```python
from build123d import *

# Parameters (mm, degrees)
F1_DEPTH = 40
F2_R     = 34
F3_T     = -1
F4_DEPTH = 1


# Not quite as in the source:
# - a shell that OpenCascade refuses in one call is made with other operations: the cavity is built on its own and cut out
# - a feature names something its author has since deleted; it is built from what else it names


with BuildPart() as f1:
    # F0 (on Top) → F1 (new body)
    with BuildSketch(Plane.XY):
        with BuildLine():
            Line((37, 0.6), (39.9954997468, 0.6))
            ThreePointArc((39.9954997468, 0.6), (28.2842712475, 28.2842712475), (0.6, 39.9954997468))
            Line((0.6, 39.9954997468), (0.6, 37))
            Line((0.6, 37), (-2.4, 37))
            Line((-2.4, 37), (-2.4, 39.9279350831))
            ThreePointArc((-2.4, 39.9279350831), (-28.9139450641, 27.6402565261), (-39.9954997468, 0.6))
            Line((-39.9954997468, 0.6), (-37, 0.6))
            Line((-37, 0.6), (-37, -2.4))
            Line((-37, -2.4), (-39.9279350831, -2.4))
            ThreePointArc((-39.9279350831, -2.4), (-28.2842712475, -28.2842712475), (-2.4, -39.9279350831))
            Line((-2.4, -39.9279350831), (-2.4, -37))
            Line((-2.4, -37), (0.6, -37))
            Line((0.6, -37), (0.6, -39.9954997468))
            ThreePointArc((0.6, -39.9954997468), (27.6402565261, -28.9139450641), (39.9279350831, -2.4))
            Line((39.9279350831, -2.4), (37, -2.4))
            Line((37, -2.4), (37, 0.6))
        make_face()
        with BuildLine():
            ThreePointArc((39.9279350831, -2.4), (39.9819797116, -1.2005408523), (40, 0))
            ThreePointArc((40, 0), (39.9988749209, 0.3000084383), (39.9954997468, 0.6))
            Line((39.9954997468, 0.6), (37, 0.6))
            Line((37, 0.6), (37, -2.4))
            Line((37, -2.4), (39.9279350831, -2.4))
        make_face()
        with BuildLine():
            Line((37, 0.6), (39.9954997468, 0.6))
            ThreePointArc((39.9954997468, 0.6), (28.2842712475, 28.2842712475), (0.6, 39.9954997468))
            Line((0.6, 39.9954997468), (0.6, 37))
            Line((0.6, 37), (-2.4, 37))
            Line((-2.4, 37), (-2.4, 39.9279350831))
            ThreePointArc((-2.4, 39.9279350831), (-28.9139450641, 27.6402565261), (-39.9954997468, 0.6))
            Line((-39.9954997468, 0.6), (-37, 0.6))
            Line((-37, 0.6), (-37, -2.4))
            Line((-37, -2.4), (-39.9279350831, -2.4))
            ThreePointArc((-39.9279350831, -2.4), (-28.2842712475, -28.2842712475), (-2.4, -39.9279350831))
            Line((-2.4, -39.9279350831), (-2.4, -37))
            Line((-2.4, -37), (0.6, -37))
            Line((0.6, -37), (0.6, -39.9954997468))
            ThreePointArc((0.6, -39.9954997468), (27.6402565261, -28.9139450641), (39.9279350831, -2.4))
            Line((39.9279350831, -2.4), (37, -2.4))
            Line((37, -2.4), (37, 0.6))
        make_face()
        with BuildLine():
            Line((37, 0.6), (39.9954997468, 0.6))
            ThreePointArc((39.9954997468, 0.6), (28.2842712475, 28.2842712475), (0.6, 39.9954997468))
            Line((0.6, 39.9954997468), (0.6, 37))
            Line((0.6, 37), (-2.4, 37))
            Line((-2.4, 37), (-2.4, 39.9279350831))
            ThreePointArc((-2.4, 39.9279350831), (-28.9139450641, 27.6402565261), (-39.9954997468, 0.6))
            Line((-39.9954997468, 0.6), (-37, 0.6))
            Line((-37, 0.6), (-37, -2.4))
            Line((-37, -2.4), (-39.9279350831, -2.4))
            ThreePointArc((-39.9279350831, -2.4), (-28.2842712475, -28.2842712475), (-2.4, -39.9279350831))
            Line((-2.4, -39.9279350831), (-2.4, -37))
            Line((-2.4, -37), (0.6, -37))
            Line((0.6, -37), (0.6, -39.9954997468))
            ThreePointArc((0.6, -39.9954997468), (27.6402565261, -28.9139450641), (39.9279350831, -2.4))
            Line((39.9279350831, -2.4), (37, -2.4))
            Line((37, -2.4), (37, 0.6))
        make_face()
        with BuildLine():
            Line((37, 0.6), (39.9954997468, 0.6))
            ThreePointArc((39.9954997468, 0.6), (28.2842712475, 28.2842712475), (0.6, 39.9954997468))
            Line((0.6, 39.9954997468), (0.6, 37))
            Line((0.6, 37), (-2.4, 37))
            Line((-2.4, 37), (-2.4, 39.9279350831))
            ThreePointArc((-2.4, 39.9279350831), (-28.9139450641, 27.6402565261), (-39.9954997468, 0.6))
            Line((-39.9954997468, 0.6), (-37, 0.6))
            Line((-37, 0.6), (-37, -2.4))
            Line((-37, -2.4), (-39.9279350831, -2.4))
            ThreePointArc((-39.9279350831, -2.4), (-28.2842712475, -28.2842712475), (-2.4, -39.9279350831))
            Line((-2.4, -39.9279350831), (-2.4, -37))
            Line((-2.4, -37), (0.6, -37))
            Line((0.6, -37), (0.6, -39.9954997468))
            ThreePointArc((0.6, -39.9954997468), (27.6402565261, -28.9139450641), (39.9279350831, -2.4))
            Line((39.9279350831, -2.4), (37, -2.4))
            Line((37, -2.4), (37, 0.6))
        make_face()
        with BuildLine():
            ThreePointArc((39.9279350831, -2.4), (39.9819797116, -1.2005408523), (40, 0))
            ThreePointArc((40, 0), (39.9988749209, 0.3000084383), (39.9954997468, 0.6))
            Line((39.9954997468, 0.6), (37, 0.6))
            Line((37, 0.6), (37, -2.4))
            Line((37, -2.4), (39.9279350831, -2.4))
        make_face()
        with BuildLine():
            ThreePointArc((-2.4, -39.9279350831), (-0.9006338024, -39.989859449), (0.6, -39.9954997468))
            Line((0.6, -39.9954997468), (0.6, -37))
            Line((0.6, -37), (-2.4, -37))
            Line((-2.4, -37), (-2.4, -39.9279350831))
        make_face()
        with BuildLine():
            Line((-37, 0.6), (-39.9954997468, 0.6))
            ThreePointArc((-39.9954997468, 0.6), (-39.989859449, -0.9006338024), (-39.9279350831, -2.4))
            Line((-39.9279350831, -2.4), (-37, -2.4))
            Line((-37, -2.4), (-37, 0.6))
        make_face()
        with BuildLine():
            Line((0.6, 37), (0.6, 39.9954997468))
            ThreePointArc((0.6, 39.9954997468), (-0.9006338024, 39.989859449), (-2.4, 39.9279350831))
            Line((-2.4, 39.9279350831), (-2.4, 37))
            Line((-2.4, 37), (0.6, 37))
        make_face()
        with BuildLine():
            Line((37, 0.6), (39.9954997468, 0.6))
            ThreePointArc((39.9954997468, 0.6), (28.2842712475, 28.2842712475), (0.6, 39.9954997468))
            Line((0.6, 39.9954997468), (0.6, 37))
            Line((0.6, 37), (-2.4, 37))
            Line((-2.4, 37), (-2.4, 39.9279350831))
            ThreePointArc((-2.4, 39.9279350831), (-28.9139450641, 27.6402565261), (-39.9954997468, 0.6))
            Line((-39.9954997468, 0.6), (-37, 0.6))
            Line((-37, 0.6), (-37, -2.4))
            Line((-37, -2.4), (-39.9279350831, -2.4))
            ThreePointArc((-39.9279350831, -2.4), (-28.2842712475, -28.2842712475), (-2.4, -39.9279350831))
            Line((-2.4, -39.9279350831), (-2.4, -37))
            Line((-2.4, -37), (0.6, -37))
            Line((0.6, -37), (0.6, -39.9954997468))
            ThreePointArc((0.6, -39.9954997468), (27.6402565261, -28.9139450641), (39.9279350831, -2.4))
            Line((39.9279350831, -2.4), (37, -2.4))
            Line((37, -2.4), (37, 0.6))
        make_face()
        with BuildLine():
            Line((37, 0.6), (39.9954997468, 0.6))
            ThreePointArc((39.9954997468, 0.6), (28.2842712475, 28.2842712475), (0.6, 39.9954997468))
            Line((0.6, 39.9954997468), (0.6, 37))
            Line((0.6, 37), (-2.4, 37))
            Line((-2.4, 37), (-2.4, 39.9279350831))
            ThreePointArc((-2.4, 39.9279350831), (-28.9139450641, 27.6402565261), (-39.9954997468, 0.6))
            Line((-39.9954997468, 0.6), (-37, 0.6))
            Line((-37, 0.6), (-37, -2.4))
            Line((-37, -2.4), (-39.9279350831, -2.4))
            ThreePointArc((-39.9279350831, -2.4), (-28.2842712475, -28.2842712475), (-2.4, -39.9279350831))
            Line((-2.4, -39.9279350831), (-2.4, -37))
            Line((-2.4, -37), (0.6, -37))
            Line((0.6, -37), (0.6, -39.9954997468))
            ThreePointArc((0.6, -39.9954997468), (27.6402565261, -28.9139450641), (39.9279350831, -2.4))
            Line((39.9279350831, -2.4), (37, -2.4))
            Line((37, -2.4), (37, 0.6))
        make_face()
    extrude(amount=F1_DEPTH)

    # F2
    f2_edges = [f1.edges().sort_by_distance(p)[0] for p in [
        (-0.6, -39.9955, 40),
    ]]
    fillet(f2_edges, radius=F2_R)

    # F3: a shell. OpenCascade refuses it in one call, so the cavity is built on its own and cut out:
    # the body offset inwards by the wall thickness, plus a prism from it out through each open face.
    f3_core = offset(f1.part, amount=F3_T, mode=Mode.PRIVATE)
    f3_exits = [f3_core.faces().sort_by_distance(p)[0] for p in [
        (0, 0, 39),
        (0, 0, 1),
    ]]
    add(f3_core, mode=Mode.SUBTRACT)
    extrude(f3_exits, amount=-F3_T, mode=Mode.SUBTRACT)

    # F0 (on Top) → F4 (join)
    with BuildSketch(Plane.XY):
        with BuildLine():
            ThreePointArc((39.9279350831, -2.4), (39.9819797116, -1.2005408523), (40, 0))
            ThreePointArc((40, 0), (39.9988749209, 0.3000084383), (39.9954997468, 0.6))
            Line((39.9954997468, 0.6), (37, 0.6))
            Line((37, 0.6), (37, -2.4))
            Line((37, -2.4), (39.9279350831, -2.4))
        make_face()
        with BuildLine():
            Line((0.6, 37), (0.6, 39.9954997468))
            ThreePointArc((0.6, 39.9954997468), (-0.9006338024, 39.989859449), (-2.4, 39.9279350831))
            Line((-2.4, 39.9279350831), (-2.4, 37))
            Line((-2.4, 37), (0.6, 37))
        make_face()
        with BuildLine():
            Line((-37, 0.6), (-39.9954997468, 0.6))
            ThreePointArc((-39.9954997468, 0.6), (-39.989859449, -0.9006338024), (-39.9279350831, -2.4))
            Line((-39.9279350831, -2.4), (-37, -2.4))
            Line((-37, -2.4), (-37, 0.6))
        make_face()
        with BuildLine():
            ThreePointArc((-2.4, -39.9279350831), (-0.9006338024, -39.989859449), (0.6, -39.9954997468))
            Line((0.6, -39.9954997468), (0.6, -37))
            Line((0.6, -37), (-2.4, -37))
            Line((-2.4, -37), (-2.4, -39.9279350831))
        make_face()
    extrude(amount=F4_DEPTH)


solid = f1.part
```
Verification items for the finished model (mm, model axes). Round coordinates to 2 decimals unless told otherwise and drop trailing zeros. Use CSV: the item, a comma, the result in double quotes. Start each with the question number.
1) Mould release check, pull along Y, two halves, no side actions. Record for faces 1 (the flat face through (0, -38, 0)), 2 (the flat face through (-1, -38, 1)): +Y half, -Y half, draft (parallel to the pull), parting line (faces both ways), or undercut.
2) Go/stop test with flat-tipped pins: P1, Ø1.1, axis at y = -37.5, z = 0.5, coming from the -X side; P2, Ø1.5, axis at y = -26, z = 29.5, coming from the +X side; P3, Ø8, axis at x = 19, z = 18.5, coming from the -Y side. Record where each tip stops, or that it passes through.
3) Thickness scan on L1, parallel to X at y = -23, z = 25.5; L2, parallel to Y at x = -15, z = 11.5; L3, parallel to Y at x = -2.5, z = 32. Record the ranges inside material, lowest first.
Answers:
1,face 1,"draft"
1,face 2,"undercut"
2,P1,"stops at x = -15.32"
2,P2,"stops at x = 17.79"
2,P3,"stops at y = -35.07"
3,L1,"x = -24.84 to -23.13, 23.13 to 24.84"
3,L2,"y = -36.6 to -35.5, 35.5 to 36.6"
3,L3,"y = -27.8 to -26.2, 26.2 to 27.8"
